For this review, take the finished solid that the model builds, in its own axes (mm). A direction names the side the tool comes from. Round coordinates to 2 decimals unless told otherwise and drop trailing zeros. Order: outer loops, then holes, each group sorted by start corner. A loop starts at its lowest first (then second) coordinate and runs counter-clockwise, first axis right, second up. Notation, with made-up numbers: M 65,87 L 90,87 A12 ccw 90,102 Z; hole C 40,13.5 d1. An arc over 180 degrees is marked long. Use a Markdown table: item, result.
from build123d import *

# Parameters (mm, degrees)
BOSS_EXTRUDE1_DEPTH                             = 47.5
CSK_FOR_M3_FLAT_HEAD_MACHINE_SCREW1_D           = 3.4
CSK_FOR_M3_FLAT_HEAD_MACHINE_SCREW1_CSINK_D     = 6.3
CSK_FOR_M3_FLAT_HEAD_MACHINE_SCREW1_CSINK_ANGLE = 90
SKETCH5_R                                       = 2.7
CUT_EXTRUDE1_DEPTH                              = 31.1


with BuildPart() as part:
    # Sketch1 → Boss-Extrude1 (new body)
    with BuildSketch(Plane(origin=(0, 0, 0), x_dir=(0, 0, -1), z_dir=(1, 0, 0))):
        Polygon((10.05, -10.05), (10.05, -15.05), (-15.05, -15.05), (-15.05, 15.05), (10.05, 15.05), (10.05, 10.05), (-10.05, 10.05), (-10.05, -10.05), align=None)
    extrude(amount=BOSS_EXTRUDE1_DEPTH)

    # CSK for M3 Flat Head Machine Screw1 (through all)
    with Locations(Plane(origin=(0, 0, 10.05), x_dir=(-1, 0, 0), z_dir=(0, 0, -1))):
        with Locations((-29.406854249, 5.656854249), (-18.093145751, 5.656854249), (-18.093145751, -5.656854249), (-29.406854249, -5.656854249)):
            CounterSinkHole(CSK_FOR_M3_FLAT_HEAD_MACHINE_SCREW1_D / 2, CSK_FOR_M3_FLAT_HEAD_MACHINE_SCREW1_CSINK_D / 2, counter_sink_angle=CSK_FOR_M3_FLAT_HEAD_MACHINE_SCREW1_CSINK_ANGLE)

    # Sketch5 → Cut-Extrude1 (cut, through all)
    with BuildSketch(Plane(origin=(0, 15.05, 0), x_dir=(1, 0, 0), z_dir=(0, 1, 0))):
        with Locations((10, 0)):
            Circle(SKETCH5_R)
        with Locations((37.5, 0)):
            Circle(SKETCH5_R)
    extrude(amount=-CUT_EXTRUDE1_DEPTH, mode=Mode.SUBTRACT)


solid = part.part
Q1. Add section C-C (z = 0). Write out the cut boundary in (x, y).
Determined:
| item | result |
|---|---|
| outline | M 0,-15.05 L 7.3,-15.05 L 7.3,-10.05 L 0,-10.05 Z; M 0,10.05 L 7.3,10.05 L 7.3,15.05 L 0,15.05 Z; M 12.7,-15.05 L 34.8,-15.05 L 34.8,-10.05 L 12.7,-10.05 Z; M 12.7,10.05 L 34.8,10.05 L 34.8,15.05 L 12.7,15.05 Z; M 40.2,-15.05 L 47.5,-15.05 L 47.5,-10.05 L 40.2,-10.05 Z; M 40.2,10.05 L 47.5,10.05 L 47.5,15.05 L 40.2,15.05 Z |
Q2. Add section B-B (z = 8.5). Write out the cut boundary in (x, y), then the cut area to 3 significant figures.
Determined:
| item | result |
|---|---|
| outline | M 0,-15.05 L 47.5,-15.05 L 47.5,-10.05 L 0,-10.05 Z; M 0,10.05 L 47.5,10.05 L 47.5,15.05 L 0,15.05 Z |
| area | 475 mm^2 |
Q3. Add section D-D (x = 5). Write out the cut boundary in (y, z), then the cut area to 4 significant figures.
Determined:
| item | result |
|---|---|
| outline | M -15.05,-10.05 L -10.05,-10.05 L -10.05,10.05 L 10.05,10.05 L 10.05,-10.05 L 15.05,-10.05 L 15.05,15.05 L -15.05,15.05 Z |
| area | 351.5 mm^2 |
Q4. Wall thickness on line 1 along X through (y, z) = (-13.45, 0); line 2 along Y through (x, z) = (9.5, -3); line 3 along X through (y, z) = (5, 13): over which ranges is each line inside the solid? List them lowest first. Write a range as [from, to].
Determined:
| item | result |
|---|---|
| line 1 | x = [0, 7.3], [12.7, 34.8], [40.2, 47.5] |
| line 2 | y = [-15.05, -10.05], [10.05, 15.05] |
| line 3 | x = [0, 16.53], [19.66, 27.84], [30.97, 47.5] |
Q5. Machinability: for faces 1 (the flat face through (23, 10.05, 0)), 2 (the cylindrical face through (40.075, 12.585, -0.811)), which of the approach directions +Z, -Z, +X, -X, +Y, -Y give a long, thin tool a straight path to every point of the face, cutting with its end or side? Answer none if there is none.
Determined:
| item | result |
|---|---|
| face 1 | -Z, +X, -X |
| face 2 | +Y, -Y |
Q6. Clearance check with flat-ended pins moving along their axes: pin 1 (2.5 mm diameter, centred on x = 29.41, y = 5.66, fed in from -Z); pin 2 (4 mm diameter, centred on x = 18.09, y = 5.66, fed in from -Z); pin 3 (5 mm diameter, centred on x = 12, y = 0, fed in from -Z). State where each tip first meets the part, or that it passes through.
Determined:
| item | result |
|---|---|
| pin 1 | passes through |
| pin 2 | stops at z = 11.2 |
| pin 3 | stops at z = 10.05 |
Q7. Add section A-A (x = 37.5). Write out the cut boundary in (y, z), then the cut area to 4 significant figures.
Determined:
| item | result |
|---|---|
| outline | M -15.05,-10.05 L -10.05,-10.05 L -10.05,-2.7 L -15.05,-2.7 Z; M -15.05,2.7 L -10.05,2.7 L -10.05,10.05 L 10.05,10.05 L 10.05,2.7 L 15.05,2.7 L 15.05,15.05 L -15.05,15.05 Z; M 10.05,-10.05 L 15.05,-10.05 L 15.05,-2.7 L 10.05,-2.7 Z |
| area | 297.5 mm^2 |
Q8. Draft analysis for pull direction X (two halves, no side actions). For faces 3 (the cylindrical face through (12.575, -12.515, -0.811)), 4 (the flat face through (23, -10.05, 0)), 5 (the flat face through (0, 4, 11)), state which applies: pulls with the +X half, pulls with the -X half, needs draft (parallel to the pull), parting line crosses it, or undercut.
Determined:
| item | result |
|---|---|
| face 3 | undercut |
| face 4 | needs draft |
| face 5 | pulls with the -X half |
